CAD build for the part. Positions are in the model's coordinates, mm. Give positions to 0.01 mm unless a question says otherwise; leave off trailing zeros. Loops run counter-clockwise (first coordinate to the right, second up) from the corner with the lowest first, then second, coordinate; pieces in that order, holes last.
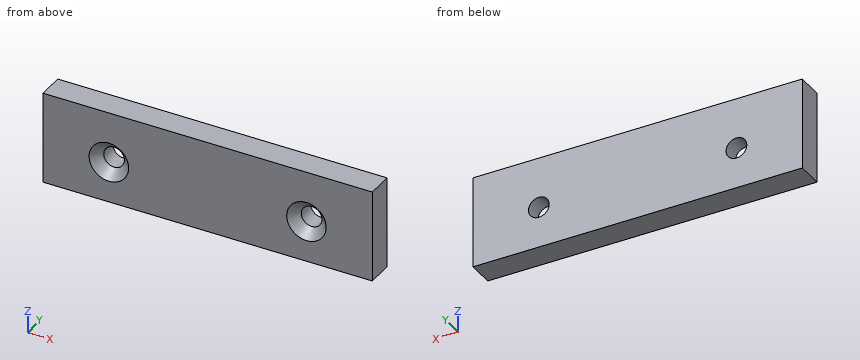
Solid Edge part; units mm, degrees
sketch "Sketch1" plane through (0, 0, 0) normal (0, -1, 0) x (1, 0, 0)
  line L0 (-50, 14) -> (50, 14)
  line L1 (50, 14) -> (50, -14)
  line L2 (50, -14) -> (-50, -14)
  line L3 (-50, -14) -> (-50, 14)
  dimension "D1" = 50
  dimension "D2" = 50
extrude "Protrusion1" add sketch "Sketch1" along normal blind 8
hole "Hole_3" at (30, -8, -1.5) direction (0, 1, 0) diameter 6.3 end up to next countersink diameter 12 countersink angle 90
hole "Hole1" at (-30, -8, -1.5) direction (0, 1, 0) diameter 6.3 end up to next countersink diameter 12 countersink angle 90
properties part number "3" material "cast iron"
1. Saw through at B-B, the plane z = -1.5. List the corners of the cut face in (x, y).
Responses:
outline: (-50, -8) - (-36, -8) - (-33.15, -5.15) - (-33.15, 0) - (-50, 0) - close; (-26.85, -5.15) - (-24, -8) - (24, -8) - (26.85, -5.15) - (26.85, 0) - (-26.85, 0) - close; (33.15, -5.15) - (36, -8) - (50, -8) - (50, 0) - (33.15, 0) - close
2. Probe line 1 along X through (y, z) = (-1.1, -1.5); line 2 along Z through (x, y) = (30, -1.5); line 3 along X through (y, z) = (-5.75, 1.75). List the from-to ranges inside material, lowest first.
Responses:
line 1: x = -50 to -33.15, -26.85 to 26.85, 33.15 to 50
line 2: z = -14 to -4.65, 1.65 to 14
line 3: x = -50 to -31.87, -28.13 to 28.13, 31.87 to 50
3. Saw through at C-C, the plane y = -3. List the corners of the cut face in (x, z).
Responses:
outline: (-50, -14) - (50, -14) - (50, 14) - (-50, 14) - close; hole circle Ø6.3 at (-30, -1.5); hole circle Ø6.3 at (30, -1.5)
4. Saw through at A-A, the plane x = -30. List the corners of the cut face in (y, z), and give its area (3 significant figures).
Responses:
outline: (-8, -14) - (0, -14) - (0, -4.65) - (-5.15, -4.65) - (-8, -7.5) - close; (-8, 4.5) - (-5.15, 1.65) - (0, 1.65) - (0, 14) - (-8, 14) - close
area: 165 mm2
5. Drop a flat-ended pin along its axis: pin 1 (4 mm diameter, centred on x = -30, z = -1.5, fed in from +Y). Give the stop position or say it passes through.
Responses:
pin 1: passes through
